Answer from the drawing. Dimensions are ordinates in mm from the lowest x, y and z of the part. Give positions to 0.01 mm unless a question says otherwise; leave off trailing zeros. Order: outer loops, then holes, each group sorted by start corner. A loop starts at its lowest first (then second) coordinate and runs counter-clockwise, first axis right, second up.
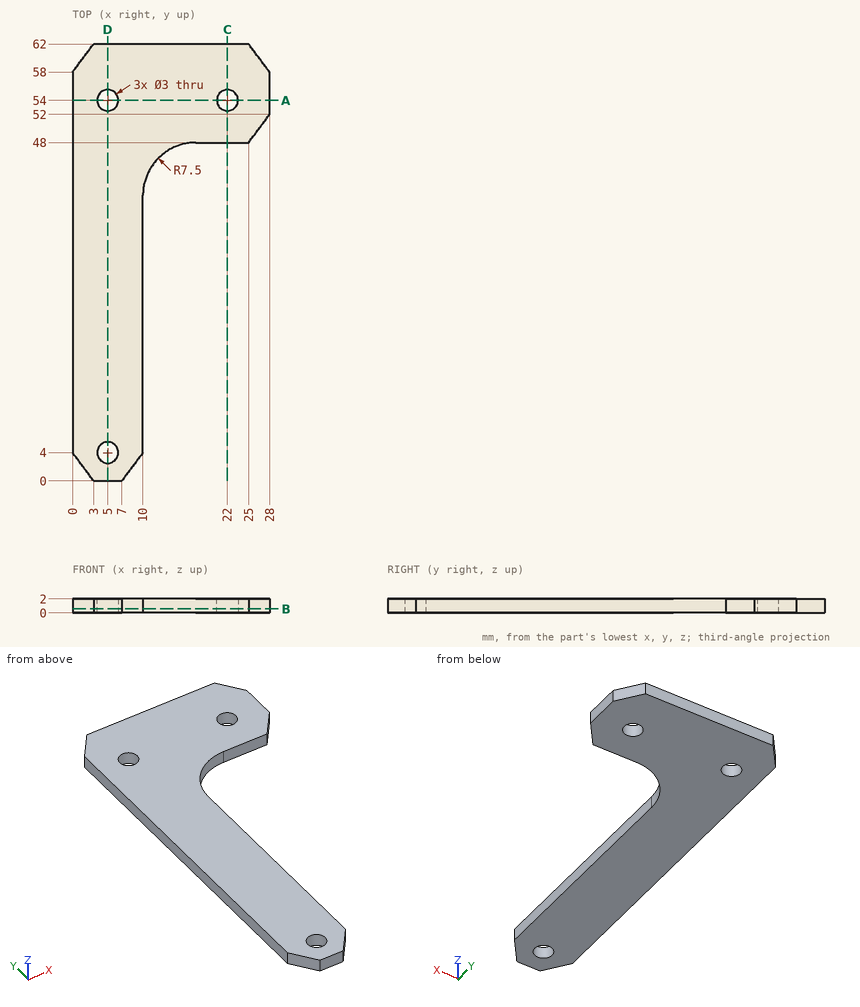
1. The part is cut by section B-B (z = 0.55). Write down the section's boundary in (x, y).
Findings below:
outline: (0, 4) - (3, 0) - (7, 0) - (10, 4) - (10, 40.5) arc R7.5 cw to (17.5, 48) - (25, 48) - (28, 52) - (28, 58) - (25, 62) - (3, 62) - (0, 58) - close; hole circle Ø3 at (5, 4); hole circle Ø3 at (5, 54); hole circle Ø3 at (22, 54)
2. The part is cut by section C-C (x = 22). Write down the section's boundary in (y, z), then the cut area to 3 significant figures.
Findings below:
outline: (48, 0) - (52.5, 0) - (52.5, 2) - (48, 2) - close; (55.5, 0) - (62, 0) - (62, 2) - (55.5, 2) - close
area: 22.0 mm2
3. The part is cut by section A-A (y = 54). Write down the section's boundary in (x, z), then the cut area to 3 significant figures.
Findings below:
outline: (0, 0) - (3.5, 0) - (3.5, 2) - (0, 2) - close; (6.5, 0) - (20.5, 0) - (20.5, 2) - (6.5, 2) - close; (23.5, 0) - (28, 0) - (28, 2) - (23.5, 2) - close
area: 44.0 mm2
4. The part is cut by section D-D (x = 5). Write down the section's boundary in (y, z), then the cut area to 3 significant figures.
Findings below:
outline: (0, 0) - (2.5, 0) - (2.5, 2) - (0, 2) - close; (5.5, 0) - (52.5, 0) - (52.5, 2) - (5.5, 2) - close; (55.5, 0) - (62, 0) - (62, 2) - (55.5, 2) - close
area: 112 mm2
5. Given P1, Ø2, axis at x = 5, y = 17.5, coming from the -Z side; P2, Ø2.5, axis at x = 5, y = 4, coming from the -Z side, each flat-ended and moving along its own axis, determine where each tip first touches the part or whether it passes through.
Findings below:
P1: stops at z = 0
P2: passes through
6. Straight lines are drawn through the part: probe 1 along Y at (x, z) = (5, 0.55); probe 2 along Y at (x, z) = (22, 1); probe 3 along X at (y, z) = (34, 0.35). For each, find the intervals that lie inside material, in ascending order.
Findings below:
probe 1: y = 0 to 2.5, 5.5 to 52.5, 55.5 to 62
probe 2: y = 48 to 52.5, 55.5 to 62
probe 3: x = 0 to 10
